The listing builds one solid part. Answer for the finished solid, in the listing's coordinates (mm). A direction names the side the tool comes from. Coordinates: 2 decimals unless noted, no trailing zeros. Order: outer loops, then holes, each group sorted by start corner. A loop starts at its lowest first (then second) coordinate and runs counter-clockwise, first axis right, second up. Notation, with made-up numbers: (89.25, 43) - (106.25, 43) arc R21 ccw to (106.25, 48) - close; hole circle Ø10 at (-38, -2). An arc over 180 degrees is marked (long way). Use a Markdown table: item, result. Add a question column.
Item 1: The mould has two halves that part along X. Classify faces 1 (the flat face through (-12.765, 7.409, -3.621)), 2 (the flat face through (-4, 7, -12)), 3 (the flat face through (-4, 15, -12)): released by +X, released by -X, zero draft, split by the parting line, or undercut.
Item 2: A flat-ended cylindrical pin translates along its axis: P1, Ø4.5, axis at x = -6.29, y = 10, coming from the -Z side. Find the tip coordinate at first contact, or state that the pin passes through.
Item 3: The part is cut by section A-A, the plane z = -19. Give the vertices of the cut face in (x, y) (3 decimals), then the cut area to 3 significant figures.
Item 4: For faces 4 (the cylindrical face through (-5.021, 3.451, -5.927)), 5 (the flat face through (-12.7, 0.7, -19.9)), determine the directions among +Z, -Z, +X, -X, +Y, -Y from which every point of the face is accessible in a straight line to the end or side of a thin tool.
Item 5: Find the intervals of material crossed by line 1 along X through (y, z) = (11.75, -18.25); line 2 along X through (y, z) = (9.5, -8.25); line 3 along Y through (x, z) = (-7.75, -7.5), in increasing order.
Item 6: The part is cut by section B-B, the plane y = 10. Give the vertices of the cut face in (x, z), then the cut area to 3 significant figures.
Item 7: The part is cut by section D-D, the plane z = -13. Give the vertices of the cut face in (x, y) (3 decimals).
Item 8: The part is cut by section C-C, the plane y = 2.75. Give the vertices of the cut face in (x, z), then the cut area to 3 significant figures.
from build123d import *

# Parameters (mm, degrees)
SKETCH1_W           = 18
SKETCH1_H           = 18
BOSS_EXTRUDE1_DEPTH = 15
SKETCH2_R           = 2.625
CUT_EXTRUDE1_DEPTH  = 19
SKETCH3_R           = 5.75
CUT_EXTRUDE2_DEPTH  = 7
SKETCH5_W           = 18
SKETCH5_H           = 15
CUT_EXTRUDE3_DEPTH  = 0.5
CHAMFER1_SIZE       = 1


with BuildPart() as part:
    # Sketch1 → Boss-Extrude1 (new body)
    with BuildSketch(Plane(origin=(0, 0, 0), x_dir=(1, 0, 0), z_dir=(0, 1, 0))):
        with Locations((-4.272296667, 11.628336988)):
            Rectangle(SKETCH1_W, SKETCH1_H)
    extrude(amount=BOSS_EXTRUDE1_DEPTH)

    # Sketch2 → Cut-Extrude1 (cut, through all)
    with BuildSketch(Plane.XY.offset(-2.628336988)):
        with Locations((-6.286796667, 10)):
            Circle(SKETCH2_R)
    extrude(amount=-CUT_EXTRUDE1_DEPTH, mode=Mode.SUBTRACT)

    # Sketch3 → Cut-Extrude2 (cut)
    with BuildSketch(Plane.XZ):
        with Locations((-4.272296667, -11.628336988)):
            Circle(SKETCH3_R)
    extrude(amount=-CUT_EXTRUDE2_DEPTH, mode=Mode.SUBTRACT)

    # Sketch5 → Cut-Extrude3 (cut)
    with BuildSketch(Plane.XY.offset(-2.628336988)):
        with Locations((-4.272296667, 7.5)):
            Rectangle(SKETCH5_W, SKETCH5_H)
    extrude(amount=-CUT_EXTRUDE3_DEPTH, mode=Mode.SUBTRACT)

    # Chamfer1
    chamfer1_edges = [part.edges().sort_by_distance(p)[0] for p in [
        (-4.272296667, 15, -20.628336988),
        (4.727703333, 0, -11.878336988),
        (4.727703333, 15, -11.878336988),
        (-4.272296667, 15, -3.128336988),
        (4.727703333, 7.5, -3.128336988),
        (-4.272296667, 0, -3.128336988),
        (-13.272296667, 7.5, -3.128336988),
        (-13.272296667, 15, -11.878336988),
        (-4.272296667, 0, -20.628336988),
        (-13.272296667, 0, -11.878336988),
        (-13.272296667, 7.5, -20.628336988),
        (4.727703333, 7.5, -20.628336988),
    ]]
    chamfer(chamfer1_edges, length=CHAMFER1_SIZE)


solid = part.part
Solution:
| question | item | result |
|---|---|---|
| 1 | face 1 | released by -X |
| 1 | face 2 | undercut |
| 1 | face 3 | zero draft |
| 2 | P1 | passes through |
| 3 | outline | (-13.272, 1) - (-12.272, 0) - (3.728, 0) - (4.728, 1) - (4.728, 14) - (3.728, 15) - (-12.272, 15) - (-13.272, 14) - close; hole circle Ø5.25 at (-6.287, 10) |
| 3 | area | 246 mm2 |
| 4 | face 4 | -Y |
| 4 | face 5 | -Z, -X, -Y |
| 5 | line 1 | x = -13.27 to -8.24, -4.33 to 4.73 |
| 5 | line 2 | x = -13.27 to -8.86, -3.71 to 4.73 |
| 5 | line 3 | y = 7 to 7.82, 12.18 to 15 |
| 6 | outline | (-13.27, -19.63) - (-12.27, -20.63) - (-8.91, -20.63) - (-8.91, -3.13) - (-12.27, -3.13) - (-13.27, -4.13) - close; (-3.66, -20.63) - (3.73, -20.63) - (4.73, -19.63) - (4.73, -4.13) - (3.73, -3.13) - (-3.66, -3.13) - close |
| 6 | area | 221 mm2 |
| 7 | outline | (-13.272, 1) - (-12.272, 0) - (-9.856, 0) - (-9.856, 7) - (1.312, 7) - (1.312, 0) - (3.728, 0) - (4.728, 1) - (4.728, 14) - (3.728, 15) - (-12.272, 15) - (-13.272, 14) - close; hole circle Ø5.25 at (-6.287, 10) |
| 8 | outline | (-13.27, -19.63) - (-12.27, -20.63) - (3.73, -20.63) - (4.73, -19.63) - (4.73, -4.13) - (3.73, -3.13) - (-12.27, -3.13) - (-13.27, -4.13) - close; hole circle Ø11.5 at (-4.27, -11.63) |
| 8 | area | 209 mm2 |
